Geometry check sheet. Reference: the model listing, model coordinates, mm. A direction names the side the tool comes from. Coordinates: 2 decimals unless noted, no trailing zeros. Loops run counter-clockwise (first coordinate to the right, second up) from the corner with the lowest first, then second, coordinate; pieces in that order, holes last. Notation, with made-up numbers: (61.25, -18.5) -> (75.25, -18.5) arc R25 ccw to (75.25, 0.5) -> close; hole circle Ø9 at (-7.5, 23). An arc over 180 degrees is marked (long way). Answer as a JSON object with one key per item and string values.
from build123d import *

# Parameters (mm, degrees)
PAD_DEPTH       = 20
POCKET_DEPTH    = 7.5
POCKET001_DEPTH = 7.5
SKETCH003_R     = 1.5
POCKET002_DEPTH = 5
SKETCH004_R     = 1.5
POCKET003_DEPTH = 5
CHAMFER_SIZE    = 1


with BuildPart() as part:
    # Sketch → Pad (new body)
    with BuildSketch(Plane.XY):
        Polygon((21.213203, 0), (0, 21.213203), (0, -21.213203), align=None)
    extrude(amount=PAD_DEPTH)

    # Sketch001 (on Face5 of Pad) → Pocket (cut)
    with BuildSketch(Plane.XY.offset(20)):
        Polygon((14.142136, 0), (0, 14.142136), (0, -14.142136), align=None)
    extrude(amount=-POCKET_DEPTH, mode=Mode.SUBTRACT)

    # Sketch002 (on Face4 of Pocket) → Pocket001 (cut)
    with BuildSketch(Plane(origin=(0, 0, 0), x_dir=(1, 0, 0), z_dir=(0, 0, -1))):
        Polygon((14.142136, 0), (0, 14.142136), (0, -14.142136), align=None)
    extrude(amount=-POCKET001_DEPTH, mode=Mode.SUBTRACT)

    # Sketch003 (on Face6 of Pocket001) → Pocket002 (cut)
    with BuildSketch(Plane(origin=(7.071068, 7.071068, 0), x_dir=(0.707107, -0.707107, 0), z_dir=(-0.707107, -0.707107, 0))):
        with Locations((-5, 16.25)):
            Circle(SKETCH003_R)
        with Locations((5, 3.75)):
            Circle(SKETCH003_R)
    extrude(amount=-POCKET002_DEPTH, mode=Mode.SUBTRACT)

    # Sketch004 (on Face10 of Pocket002) → Pocket003 (cut)
    with BuildSketch(Plane(origin=(7.071068, -7.071068, 0), x_dir=(-0.707107, -0.707107, 0), z_dir=(-0.707107, 0.707107, 0))):
        with Locations((-5, 16.25)):
            Circle(SKETCH004_R)
        with Locations((5, 3.75)):
            Circle(SKETCH004_R)
    extrude(amount=-POCKET003_DEPTH, mode=Mode.SUBTRACT)

    # Chamfer
    chamfer_edges = [part.edges().sort_by_distance(p)[0] for p in [
        (11.667262, -2.474874, 16.25),
        (9.545942, 4.596194, 3.75),
        (4.596194, -9.545942, 3.75),
        (2.474874, 11.667262, 16.25),
    ]]
    chamfer(chamfer_edges, length=CHAMFER_SIZE)


solid = part.part
1. Depth check by flat-ended pin: P1, Ø6, axis at y = 12.5, z = 6.5, coming from the +X side; P2, Ø8, axis at x = 7.5, z = 15.5, coming from the +Y side; P3, Ø4, axis at x = 5, y = 3, coming from the -Z side; P4, Ø10, axis at x = 17, y = 15.5, coming from the -Z side. Enter the tip coordinate at first touch or a pass-through.
Evaluation:
{"P1": "stops at x = 11.71", "P2": "stops at y = 17.71", "P3": "stops at z = 7.5", "P4": "passes through"}
2. Mould release check, pull along X, two halves, no side actions. Record for faces 1 (the face through (11.65, 6.7, 3.82)), 2 (the face through (10.755, 10.458, 9.86)), 3 (the face through (11.3, 3.2, 20)), 4 (the face through (0, 0, 10)): released by +X, released by -X, zero draft, split by the parting line, or undercut.
Evaluation:
{"face 1": "undercut", "face 2": "released by +X", "face 3": "zero draft", "face 4": "released by -X"}
3. Section check D-D, the plane y = -17. Record the boundary of the cut face in (x, z), then the cut area to 3 significant figures.
Evaluation:
{"outline": "(0, 0) -> (4.21, 0) -> (4.21, 20) -> (0, 20) -> close", "area": "84.3 mm^2"}
4. Tool access check on faces 5 (the face through (5, 0, 7.5)), 6 (the face through (10.458, -10.755, 9.86)), 7 (the face through (5, 0, 12.5)). Record the directions out of +Z, -Z, +X, -X, +Y, -Y that give a thin tool (end or side, any length) a straight path to the whole face; none if there is none.
Evaluation:
{"face 5": "-Z, -X", "face 6": "+Z, -Z, +X, -Y", "face 7": "+Z, -X"}
5. Section check C-C, the plane z = 17.25. State how many separate pieces and enclosed holes the cut face has, then the cut area to 3 significant figures.
Evaluation:
{"separate pieces": "3", "enclosed holes": "0", "area": "225 mm^2"}
6. Section check B-B, the plane x = 18. Record the boundary of the cut face in (y, z), then the cut area to 3 significant figures.
Evaluation:
{"outline": "(-3.21, 0) -> (3.21, 0) -> (3.21, 20) -> (-3.21, 20) -> close", "area": "129 mm^2"}
7. Section check A-A, the plane z = 11.5. Record the boundary of the cut face in (x, y).
Evaluation:
{"outline": "(0, -21.21) -> (21.21, 0) -> (0, 21.21) -> close"}
8. Thickness scan on probe 1 along Z at (x, y) = (6.25, 3.5); probe 2 along Y at (x, z) = (13.75, 6.5); probe 3 along Y at (x, z) = (3, 14.75). Record the ranges inside material, lowest first. Write a range as from..to.
Evaluation:
{"probe 1": "z = 7.5..12.5", "probe 2": "y = -7.46..-0.39, 0.39..7.46", "probe 3": "y = -18.21..-11.14, 11.89..18.21"}
